```python
from build123d import *

# Parameters (mm, degrees)
SKETCH_218_W              = 2.54
SKETCH_218_H              = 2.4
EXTRUDE_695_DEPTH         = 6.7
EXTRUDE_695_DEPTH_BACK    = 0.4
SKETCH_749_W              = 2.54
SKETCH_749_H              = 0.75
EXTRUDE_1128_DEPTH        = 0.4
SKETCH_1182_W             = 2.54
SKETCH_1182_H             = 2.4
SKETCH_1182_W_2           = 0.9
SKETCH_1182_H_2           = 0.9
EXTRUDE_1467_DEPTH        = 0.8
CHAMFER_1528_SIZE         = 0.6
PATTERN_LINEAR_1654_COUNT = 4
PATTERN_LINEAR_1654_PITCH = 2.54
EXTRUDE_1_DEPTH           = 0.64
EXTRUDE_START             = -10.8
EXTRUDE_2_DEPTH           = 0.64


with BuildPart() as part:
    # Sketch 218 → Extrude 695 (new body, two sides)
    with BuildSketch(Plane.XY) as extrude_695_sk:
        Rectangle(SKETCH_218_W, SKETCH_218_H)
        Polygon((-1, 0.35), (-0.45, 0.35), (-0.45, 0.45), (0.45, 0.45), (0.45, 0.35), (1, 0.35), (1, -0.35), (0.45, -0.35), (0.45, -0.45), (-0.45, -0.45), (-0.45, -0.35), (-1, -0.35), align=None, mode=Mode.SUBTRACT)
    extrude(amount=EXTRUDE_695_DEPTH)
    extrude(extrude_695_sk.sketch, amount=-EXTRUDE_695_DEPTH_BACK)

    # Sketch 749 → Extrude 1128 (add)
    with BuildSketch(Plane(origin=(0, 0, -0.4), x_dir=(-1, 0, 0), z_dir=(0, 0, -1))):
        with Locations((0, -0.825)):
            Rectangle(SKETCH_749_W, SKETCH_749_H)
        with Locations((0, 0.825)):
            Rectangle(SKETCH_749_W, SKETCH_749_H)
    extrude(amount=EXTRUDE_1128_DEPTH)

    # Sketch 1182 → Extrude 1467 (add)
    with BuildSketch(Plane.XY.offset(6.7)):
        Rectangle(SKETCH_1182_W, SKETCH_1182_H)
        Rectangle(SKETCH_1182_W_2, SKETCH_1182_H_2, mode=Mode.SUBTRACT)
    extrude(amount=EXTRUDE_1467_DEPTH)

    # Chamfer 1528
    chamfer_1528_edges = [part.edges().sort_by_distance(p)[0] for p in [
        (0.45, 0, 7.5),
        (0, 0.45, 7.5),
        (-0.45, 0, 7.5),
        (0, -0.45, 7.5),
    ]]
    chamfer(chamfer_1528_edges, length=CHAMFER_1528_SIZE)


with BuildPart() as pattern_linear_1654_1:
    # Pattern Linear 1654: pattern copy
    add(part.part.moved(Location(Vector(-1, 0, 0) * (1 * PATTERN_LINEAR_1654_PITCH))))


with BuildPart() as pattern_linear_1654_2:
    # Pattern Linear 1654: pattern copy
    add(part.part.moved(Location(Vector(-1, 0, 0) * (2 * PATTERN_LINEAR_1654_PITCH))))


with BuildPart() as pattern_linear_1654_3:
    # Pattern Linear 1654: pattern copy
    add(part.part.moved(Location(Vector(-1, 0, 0) * (3 * PATTERN_LINEAR_1654_PITCH))))


with BuildPart() as part_1:
    add(part.part)

    # Combine 1770: union Pattern Linear 1654_3, Pattern Linear 1654_2, Pattern Linear 1654_1
    add(pattern_linear_1654_3.part)
    add(pattern_linear_1654_2.part)
    add(pattern_linear_1654_1.part)

    # Sketch 2578 → Бобышка-БоковаяНакладка1 (add)
    with BuildSketch(Plane(origin=(1.27, 0, 0), x_dir=(0, 0, -1), z_dir=(1, 0, 0))):
        Polygon((0.8, 1.2), (0.8, 0.45), (0.4, 0.45), (0.4, -0.45), (0.8, -0.45), (0.8, -1.2), (-7.5, -1.2), (-7.5, 1.2), align=None)
    extrude(amount=EXTRUDE_1_DEPTH)

    # Эскиз-БоковаяНакладка<2> → Бобышка-БоковаяНакладка2 (add)
    with BuildSketch(Plane(origin=(1.27, 0, 0), x_dir=(0, 0, -1), z_dir=(1, 0, 0)).offset(EXTRUDE_START)):
        Polygon((0.8, 1.2), (0.8, 0.45), (0.4, 0.45), (0.4, -0.45), (0.8, -0.45), (0.8, -1.2), (-7.5, -1.2), (-7.5, 1.2), align=None)
    extrude(amount=EXTRUDE_2_DEPTH)


solid = part_1.part
```
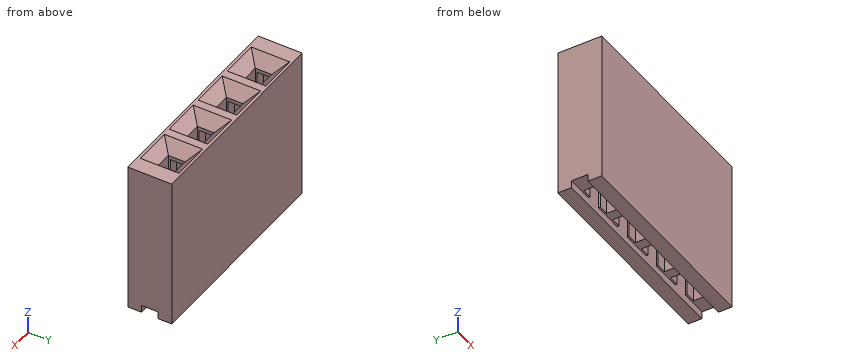
Verification items for the finished model (mm, model axes). Coordinates: 2 decimals unless noted, no trailing zeros. Write each loop counter-clockwise with the first axis right and the second up, starting at its lowest first coordinate (ties: lowest second). Pieces come first, ordered by that corner, then holes. Notation, with made-up numbers: M 72.5,14.25 L 109.5,14.25 A24 ccw 109.5,50.25 Z; hole C 18.25,70.5 d1. An arc over 180 degrees is marked long. Answer as a JSON object with one key per item and string values. Group by question number.
(1) Cross-section at B-B, the plane y = -0.6. Record the cut outline in (x, z), and give its area (3 significant figures).
(2) Cross-section at D-D, the plane z = 6.5. State how many separate pieces and enclosed holes the cut face has, and give its area (3 significant figures).
(3) Cross-section at C-C, the plane x = -4.5. Record the cut outline in (y, z), and give its area (3 significant figures).
(4) Cross-section at A-A, the plane x = 0. Record the cut outline in (y, z), and give its area (3 significant figures).
(5) Material ranges on line 1 (X direction, y = 0.2, z = 4.25); line 2 (X direction, y = 0.4, z = 0.25); line 3 (Y direction, x = -5, z = 4), recorded low to high.
(6) Gauge pin test, flat end, axial feed: pin 1 (0.7 mm diameter, centred on x = -8.5, y = 0, fed in from -Z). Record the tip position at first contact, or that the pin passes through.
Reply:
{
 "1": {"outline": "M -9.53,-0.8 L 1.91,-0.8 L 1.91,7.5 L 1.05,7.5 L 0.6,7.05 L -0.6,7.05 L -1.05,7.5 L -1.49,7.5 L -1.94,7.05 L -3.14,7.05 L -3.59,7.5 L -4.03,7.5 L -4.48,7.05 L -5.68,7.05 L -6.13,7.5 L -6.57,7.5 L -7.02,7.05 L -8.22,7.05 L -8.67,7.5 L -9.53,7.5 Z", "area": "92.0 mm²"},
 "2": {"separate pieces": "1", "enclosed holes": "4", "area": "21.1 mm²"},
 "3": {"outline": "M -1.2,-0.8 L -0.45,-0.8 L -0.45,-0.4 L -0.35,-0.4 L -0.35,6.7 L 0.35,6.7 L 0.35,-0.4 L 0.45,-0.4 L 0.45,-0.8 L 1.2,-0.8 L 1.2,7.5 L 1.05,7.5 L 0.58,7.03 L -0.58,7.03 L -1.05,7.5 L -1.2,7.5 Z", "area": "13.8 mm²"},
 "4": {"outline": "M -1.2,-0.8 L -0.45,-0.8 L -0.45,6.9 L -1.05,7.5 L -1.2,7.5 Z; M 0.45,-0.8 L 1.2,-0.8 L 1.2,7.5 L 1.05,7.5 L 0.45,6.9 Z", "area": "12.1 mm²"},
 "5": {"line 1": "-9.53 to -8.62, -6.62 to -6.08, -4.08 to -3.54, -1.54 to -1, 1 to 1.91", "line 2": "-9.53 to -8.07, -7.17 to -5.53, -4.63 to -2.99, -2.09 to -0.45, 0.45 to 1.91", "line 3": "-1.2 to -0.45, 0.45 to 1.2"},
 "6": {"pin 1": "z = -0.4"}
}
